Autodesk Inventor part; units mm, degrees
ref_plane "YZ Plane" through (0, 0, 0) normal (1, 0, 0) x (0, 1, 0)
ref_plane "XZ Plane" through (0, 0, 0) normal (0, 1, 0) x (-1, 0, 0)
ref_plane "XY Plane" through (0, 0, 0) normal (0, 0, 1) x (1, 0, 0)
sketch "Sketch1" plane through (0, 0, 0) normal (0, 1, 0) x (-1, 0, 0)
  line L0 (350, 350) -> (-350, 350)
  line L1 (-350, 350) -> (-350, -350)
  line L2 (-350, -350) -> (350, -350)
  line L3 (350, -350) -> (350, 350)
  line L4 (350, 350) -> (-350, -350) construction
  line L5 (-350, 350) -> (350, -350) construction
  line L6 (-329, 350) -> (-329, 329)
  line L7 (-329, 329) -> (-350, 329)
  line L8 (-350, -329) -> (-329, -329)
  line L9 (-329, -329) -> (-329, -350)
  line L10 (329, -350) -> (329, -329)
  line L11 (329, -329) -> (350, -329)
  line L12 (350, 329) -> (329, 329)
  line L13 (329, 329) -> (329, 350)
  line L14 (-350, 251) -> (-329, 251)
  line L15 (-329, 251) -> (-329, 251)
  line L16 (-329, 209) -> (-350, 209)
  line L17 (-329, 209) -> (-329, 251)
  line L18 (350, 0) -> (-350, 0) construction
  line L19 (0, -350) -> (0, 350) construction
  line L20 (-350, -251) -> (-329, -251)
  line L21 (-329, -209) -> (-350, -209)
  line L22 (-329, -209) -> (-329, -251)
  line L23 (0, 350) -> (0, -350) construction
  line L24 (350, 251) -> (329, 251)
  line L25 (329, 251) -> (329, 251)
  line L26 (329, 209) -> (350, 209)
  line L27 (329, 209) -> (329, 251)
  line L28 (329, -209) -> (350, -209)
  line L29 (329, -209) -> (329, -251)
  line L30 (350, -251) -> (329, -251)
  line L31 (-350, 340) -> (350, 340) construction
  circle A0 centre (262.5, 340) radius 2
  circle A1 centre (175, 340) radius 2
  circle A2 centre (87.5, 340) radius 2
  circle A3 centre (0, 340) radius 2
  circle A4 centre (-262.5, 340) radius 2
  circle A5 centre (-175, 340) radius 2
  circle A6 centre (-87.5, 340) radius 2
  line L32 (-340, -350) -> (-340, 350) construction
  circle A7 centre (-340, -175) radius 2
  circle A8 centre (-340, 0) radius 2
  circle A9 centre (-340, 87.5) radius 2
  circle A10 centre (-340, -87.5) radius 2
  circle A11 centre (-340, -262.5) radius 2
  circle A12 centre (-340, 175) radius 2
  circle A13 centre (-340, 262.5) radius 2
  line L33 (350, -340) -> (-350, -340) construction
  circle A14 centre (175, -340) radius 2
  circle A15 centre (0, -340) radius 2
  circle A16 centre (-87.5, -340) radius 2
  circle A17 centre (87.5, -340) radius 2
  circle A18 centre (262.5, -340) radius 2
  circle A19 centre (-175, -340) radius 2
  circle A20 centre (-262.5, -340) radius 2
  line L34 (340, 350) -> (340, -350) construction
  circle A21 centre (340, 175) radius 2
  circle A22 centre (340, 0) radius 2
  circle A23 centre (340, -87.5) radius 2
  circle A24 centre (340, 87.5) radius 2
  circle A25 centre (340, 262.5) radius 2
  circle A26 centre (340, -175) radius 2
  circle A27 centre (340, -262.5) radius 2
  line L35 (350, 220) -> (-350, 220) construction
  line L36 (350, 280) -> (-350, 280) construction
  circle A28 centre (262.5, 220) radius 2
  circle A29 centre (175, 220) radius 2
  circle A30 centre (87.5, 220) radius 2
  circle A31 centre (0, 220) radius 2
  circle A32 centre (-262.5, 220) radius 2
  circle A33 centre (-175, 220) radius 2
  circle A34 centre (-87.5, 220) radius 2
  circle A35 centre (175, -220) radius 2
  circle A36 centre (262.5, -220) radius 2
  circle A37 centre (-262.5, -220) radius 2
  circle A38 centre (-175, -220) radius 2
  circle A39 centre (87.5, -220) radius 2
  circle A40 centre (-87.5, -220) radius 2
  circle A41 centre (0, -220) radius 2
  line L37 (12.5, 160) -> (-12.5, 160)
  line L38 (-12.5, 160) -> (-12.5, 210)
  line L39 (-12.5, 210) -> (12.5, 210)
  line L40 (12.5, 210) -> (12.5, 160)
  line L41 (12.5, 160) -> (-12.5, 210) construction
  line L42 (-12.5, 160) -> (12.5, 210) construction
  line L43 (12.5, -160) -> (-12.5, -160)
  line L44 (-12.5, -160) -> (-12.5, -210)
  line L45 (-12.5, -210) -> (12.5, -210)
  line L46 (12.5, -210) -> (12.5, -160)
  point P0 (0, 0)
  point P1 (0, 0)
  point P2 (-350, -209)
  point P3 (350, -209)
  point P4 (350, 209)
  point P5 (0, 185)
  dimension "d0" = 700
  dimension "d1" = 700
  dimension "d2" = 21
  dimension "d3" = 21
  dimension "d6" = 360
  dimension "d8" = 21
  dimension "d9" = 99
  dimension "d10" = 141
  dimension "d13" = 10
  dimension "d14" = 4
  dimension "d15" = 4
  dimension "d16" = 4
  dimension "d17" = 175
  dimension "d18" = 87.5
  dimension "d19" = 87.5
  dimension "d20" = 4
  dimension "d23" = 360
  dimension "d25" = 130
  dimension "d26" = 120
  dimension "d27" = 60
  dimension "d28" = 140
  dimension "d29" = 25
  dimension "d30" = 50
extrude "Extrusion1" add sketch "Sketch1" along normal blind 8 contours L13 L12 L3 L24 L27 L26 L28 L29 L30 L11 L10 L2 L9 L8 L1 L20 L22 L21 L16 L17 L14 L7 L6 L0
equation "\"d1\" = d0"
equation "\"d3\" = d2"
equation "\"d15\" = d14"
equation "\"d16\" = d14"
equation "\"d18\" = 0.5 * d17"
equation "\"d19\" = d18"
equation "\"d20\" = d14"
equation "\"d27\" = 0.5 * d26"
properties part number "Bottom_Plate" material "Bamboo"
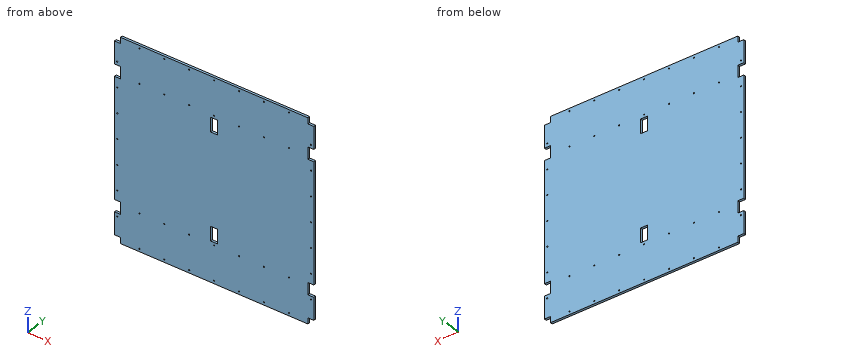
Input: part model. Units: mm. Frame: model coordinates. Round coordinates to 2 decimals unless told otherwise and drop trailing zeros.
1) Material intervals for line 1 (Z direction, x = -175, y = 3.25); line 2 (X direction, y = 3.75, z = 190.5); line 3 (X direction, y = 7, z = 242.5), sorted ascending.
Ans:
line 1: z = -350 to -342, -338 to -222, -218 to 218, 222 to 338, 342 to 350
line 2: x = -350 to -12.5, 12.5 to 350
line 3: x = -329 to 329
2) Pin query (flat end, axial travel): pin 1 (4 mm diameter, centred on y = 4.5, z = -334.5, fed in from +X); pin 2 (5 mm diameter, centred on x = 87.5, z = -340, fed in from -Y). Return the tip coordinate at first contact, or that it passes through.
Ans:
pin 1: stops at x = 329
pin 2: stops at y = 0
3) Section query A-A on y = 5.75. Count the separate pieces of the cut face and the enclosed holes in it, plus the area to 3 significant figures.
Ans:
separate pieces: 1
enclosed holes: 44
area: 482,000 mm2
